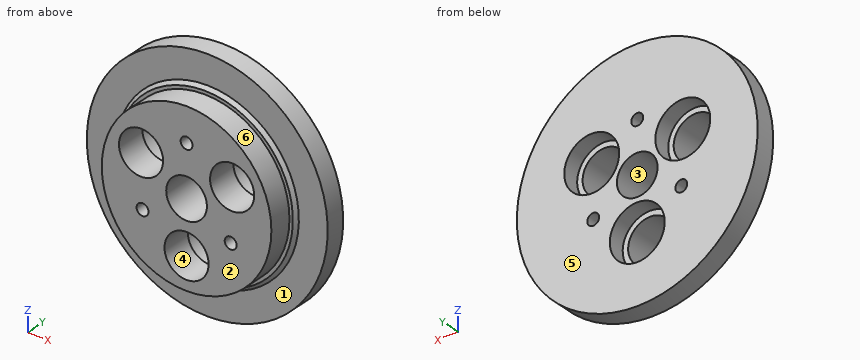
from build123d import *

# Parameters (mm, degrees)
SKETCH1_R               = 35.5
BOSS_EXTRUDE1_DEPTH     = 3
SKETCH2_R               = 26
BOSS_EXTRUDE2_DEPTH     = 1
SKETCH3_R               = 25
BOSS_EXTRUDE3_DEPTH     = 19
SKETCH5_R               = 6
CUT_EXTRUDE2_DEPTH      = 57.53759811
SKETCH6_R               = 30.018937713
SKETCH6_R_2             = 20
CUT_EXTRUDE3_DEPTH      = 12
CHAMFER2_SIZE           = 2.5
BOSS_EXTRUDE4_START     = 8
SKETCH8_R               = 25
BOSS_EXTRUDE4_DEPTH     = 8
SKETCH10_R              = 6
CUT_EXTRUDE6_DEPTH      = 61.634148794
SKETCH7_R               = 1.75
CUT_EXTRUDE4_DEPTH      = 61.634148794
BOSS_EXTRUDE5_START     = 1
SKETCH11_R              = 26
SKETCH11_R_2            = 25
BOSS_EXTRUDE5_DEPTH     = 1
CHAMFER1_SIZE           = 1
CUT_EXTRUDE7_DEPTH      = 56.222278113
CUT_EXTRUDE7_DEPTH_BACK = 56.222278113
SKETCH12_W              = 92.25680519
SKETCH12_H              = 27.524612869
SKETCH14_R              = 8.1
CUT_EXTRUDE8_DEPTH      = 5
SKETCH15_R              = 6.5
CUT_EXTRUDE9_DEPTH      = 52.004901725


with BuildPart() as part:
    # Sketch1 → Boss-Extrude1 (new, symmetric)
    with BuildSketch(Plane(origin=(0, 0, 0), x_dir=(1, 0, 0), z_dir=(0, 1, 0))):
        with Locations(Location((0, 0, 0), (0, 0, 270))):
            Circle(SKETCH1_R)
    extrude(amount=BOSS_EXTRUDE1_DEPTH, both=True)

    # Sketch2 → Boss-Extrude2 (add)
    with BuildSketch(Plane(origin=(0, 3, 0), x_dir=(1, 0, 0), z_dir=(0, 1, 0))):
        with Locations(Location((0, 0, 0), (0, 0, 270))):
            Circle(SKETCH2_R)
    extrude(amount=BOSS_EXTRUDE2_DEPTH)

    # Sketch3 → Boss-Extrude3 (add)
    with BuildSketch(Plane(origin=(0, 4, 0), x_dir=(1, 0, 0), z_dir=(0, 1, 0))):
        with Locations(Location((0, 0, 0), (0, 0, 270))):
            Circle(SKETCH3_R)
    extrude(amount=BOSS_EXTRUDE3_DEPTH)

    # Sketch5 → Cut-Extrude2 (cut, through all)
    with BuildSketch(Plane(origin=(0, 23, 0), x_dir=(1, 0, 0), z_dir=(0, 1, 0))):
        with Locations(Location((0, 0, 0), (0, 0, 270))):
            Circle(SKETCH5_R)
    extrude(amount=-CUT_EXTRUDE2_DEPTH, mode=Mode.SUBTRACT)

    # Sketch6 → Cut-Extrude3 (cut)
    with BuildSketch(Plane(origin=(0, 23, 0), x_dir=(1, 0, 0), z_dir=(0, 1, 0))):
        Circle(SKETCH6_R)
        with Locations(Location((0, 0, 0), (0, 0, 270))):
            Circle(SKETCH6_R_2, mode=Mode.SUBTRACT)
    extrude(amount=-CUT_EXTRUDE3_DEPTH, mode=Mode.SUBTRACT)

    # Chamfer2
    chamfer2_edges = [part.edges().sort_by_distance(p)[0] for p in [
        (0, 11, -20),
    ]]
    chamfer(chamfer2_edges, length=CHAMFER2_SIZE)

    # Sketch8 → Boss-Extrude4 (add)
    with BuildSketch(Plane.XZ.offset(3).offset(BOSS_EXTRUDE4_START)):
        with Locations(Location((0, 0, 0), (0, 0, 90))):
            Circle(SKETCH8_R)
    extrude(amount=-BOSS_EXTRUDE4_DEPTH)

    # Sketch10 → Cut-Extrude6 (cut, through all)
    with BuildSketch(Plane.XZ.offset(11)):
        with Locations(Location((0, 0, 0), (0, 0, 90))):
            Circle(SKETCH10_R)
    extrude(amount=-CUT_EXTRUDE6_DEPTH, mode=Mode.SUBTRACT)

    # Sketch7 → Cut-Extrude4 (cut, through all)
    with BuildSketch(Plane(origin=(0, 23, 0), x_dir=(1, 0, 0), z_dir=(0, 1, 0))):
        with Locations(Location((0, -15, 0), (0, 0, 270))):
            Circle(SKETCH7_R)
        with Locations(Location((-12.990381057, 7.5, 0), (0, 0, 270))):
            Circle(SKETCH7_R)
        with Locations(Location((12.990381057, 7.5, 0), (0, 0, 270))):
            Circle(SKETCH7_R)
    extrude(amount=-CUT_EXTRUDE4_DEPTH, mode=Mode.SUBTRACT)

    # Sketch11 → Boss-Extrude5 (add)
    with BuildSketch(Plane.XZ.offset(3).offset(BOSS_EXTRUDE5_START)):
        with Locations(Location((0, 0, 0), (0, 0, 90))):
            Circle(SKETCH11_R)
        with Locations(Location((0, 0, 0), (0, 0, 90))):
            Circle(SKETCH11_R_2, mode=Mode.SUBTRACT)
    extrude(amount=-BOSS_EXTRUDE5_DEPTH)

    # Chamfer1
    chamfer1_edges = [part.edges().sort_by_distance(p)[0] for p in [
        (0, 3, -26),
        (0, -3, -26),
    ]]
    chamfer(chamfer1_edges, length=CHAMFER1_SIZE - 0.0001)  # a hair under: the kernel refuses the full size

    # Sketch12 → Cut-Extrude7 (cut, two sides: drawn at the far end of the back side and taken through both)
    with BuildSketch(Plane.XY.offset(-CUT_EXTRUDE7_DEPTH_BACK)):
        with Locations((2.130775151, 16.762306435)):
            Rectangle(SKETCH12_W, SKETCH12_H)
    extrude(amount=CUT_EXTRUDE7_DEPTH + CUT_EXTRUDE7_DEPTH_BACK, mode=Mode.SUBTRACT)

    # Sketch14 → Cut-Extrude8 (cut)
    with BuildSketch(Plane(origin=(0, 3, 0), x_dir=(1, 0, 0), z_dir=(0, 1, 0))):
        with Locations(Location((0, 15.5, 0), (0, 0, 270))):
            Circle(SKETCH14_R)
        with Locations(Location((13.423393759, -7.75, 0), (0, 0, 270))):
            Circle(SKETCH14_R)
        with Locations(Location((-13.423393759, -7.75, 0), (0, 0, 270))):
            Circle(SKETCH14_R)
    extrude(amount=-CUT_EXTRUDE8_DEPTH, mode=Mode.SUBTRACT)

    # Sketch15 → Cut-Extrude9 (cut, through all)
    with BuildSketch(Plane(origin=(0, -2, 0), x_dir=(1, 0, 0), z_dir=(0, 1, 0))):
        with Locations(Location((0, 15.5, 0), (0, 0, 270))):
            Circle(SKETCH15_R)
        with Locations(Location((13.423393759, -7.75, 0), (0, 0, 270))):
            Circle(SKETCH15_R)
        with Locations(Location((-13.423393759, -7.75, 0), (0, 0, 270))):
            Circle(SKETCH15_R)
    extrude(amount=-CUT_EXTRUDE9_DEPTH, mode=Mode.SUBTRACT)


solid = part.part
Here's how the part is built. I have some questions about the finished solid (model axes, mm). Face numbers are marked on the shaded views. A direction names the side the tool comes from. Coordinates: 2 decimals unless noted, no trailing zeros. Write each loop counter-clockwise with the first axis right and the second up, starting at its lowest first coordinate (ties: lowest second). Pieces come first, ordered by that corner, then holes. Notation, with made-up numbers: (-13.5, 16) - (45.5, 16) arc R28 ccw to (45.5, 43) - close; hole circle Ø6 at (-0.5, 5.5). An arc over 180 degrees is marked (long way). Use one line per item in the form item = value.
1) Thinking about a two-plate mould opening in Z: for the marked faces 3, 4, 5 and 6, which applies, released by +Z, released by -Z, zero draft, split by the parting line, or undercut?
Solved:
face_3 = undercut
face_4 = undercut
face_5 = zero draft
face_6 = split by the parting line
2) Suppose I cut it at B-B, the plane y = -7.75. Write out the boundary of the cut face in (x, z), plus the area to 3 significant figures.
Solved:
outline = circle Ø50 at (0, 0); hole circle Ø13 at (-13.42, 7.75); hole circle Ø3.5 at (-12.99, -7.5); hole circle Ø13 at (0, -15.5); hole circle Ø12 at (0, 0); hole circle Ø3.5 at (0, 15); hole circle Ø13 at (13.42, 7.75); hole circle Ø3.5 at (12.99, -7.5)
area = 1,420 mm2
3) I'm going to push flat-ended pins straight in: P1, Ø8, axis at x = 16, z = 10, coming from the +Y side; P2, Ø1, axis at y = -1.5, z = 11.5, coming from the +X side; P3, Ø6, axis at y = -4.5, z = -28, coming from the +X side. Where does each tip first touch, or does it pass through?
Solved:
P1 = -2
P2 = 33.75
P3 = 24.8
4) Suppose I cut it at A-A, the plane x = 0. Give the number of separate pieces and of enclosed holes in the cut face, plus the area to 3 significant figures.
Solved:
separate_pieces = 4
enclosed_holes = 0
area = 414 mm2
5) I need wall thicknesses on line 1 (X direction, y = -5.25, z = 0); line 2 (X direction, y = -1, z = 12); line 3 (X direction, y = 0.25, z = -7). Which ranges of each line are inside material? Lowest first, please.
Solved:
line_1 = -25 to -6, 6 to 25
line_2 = -33.41 to -20.32, -6.53 to 6.53, 20.32 to 33.41
line_3 = -34.8 to -14.67, -11.31 to 11.31, 14.67 to 34.8
6) On a 3-axis mill with a long thin cutter (end or side, diameter ignored), from which of +Z, -Z, +X, -X, +Y, -Y can I reach the whole of each face in a straight line? I mean the marked faces 1 and 2. Say none if no direction works.
Solved:
face_1 = -Y
face_2 = +Z, -Z, +X, -X, -Y
7) Suppose I cut it at D-D, the plane z = 29. Write out the boundary of the cut face in (x, y).
Solved:
outline = (-20.48, -3) - (20.48, -3) - (20.48, 3) - (-20.48, 3) - close
